Verification items for the finished model (mm, model axes). A direction names the side the tool comes from. Give positions to 0.01 mm unless a question says otherwise; leave off trailing zeros. Loops run counter-clockwise (first coordinate to the right, second up) from the corner with the lowest first, then second, coordinate; pieces in that order, holes last. Notation, with made-up numbers: M 5.25,-30.75 L 59.25,-30.75 A23 ccw 59.25,-6.75 Z; hole C -12.5,-36.75 d5. An arc over 180 degrees is marked long. Use a Markdown table: item, result.
from build123d import *

# Parameters (mm, degrees)
SKETCH1_W           = 88
SKETCH1_H           = 40
BOSS_EXTRUDE1_DEPTH = 3.175
CUT_EXTRUDE1_REACH  = 5.175
SKETCH2_W           = 16
SKETCH2_H           = 3.175
SKETCH2_W_2         = 8
CUT_EXTRUDE2_REACH  = 5.175
SKETCH3_W           = 3.175
SKETCH3_H           = 8
CUT_EXTRUDE3_REACH  = 5.175
SKETCH4_R           = 2.5
CUT_EXTRUDE4_REACH  = 5.175
SKETCH5_R           = 2.5


with BuildPart() as part:
    # Sketch1 → Boss-Extrude1 (new body)
    with BuildSketch(Plane(origin=(0, 0, 0), x_dir=(1, 0, 0), z_dir=(0, 1, 0))):
        with Locations((44, -20)):
            Rectangle(SKETCH1_W, SKETCH1_H)
    extrude(amount=BOSS_EXTRUDE1_DEPTH)

    # Sketch2 → Cut-Extrude1 (cut, up to next)
    with BuildSketch(Plane(origin=(0, 3.175, 0), x_dir=(1, 0, 0), z_dir=(0, 1, 0)), mode=Mode.PRIVATE) as cut_extrude1_sk1:
        with Locations((8, -1.5875)):
            Rectangle(SKETCH2_W, SKETCH2_H)
    cut_extrude1_tool1 = extrude(cut_extrude1_sk1.sketch, amount=-CUT_EXTRUDE1_REACH, mode=Mode.PRIVATE) & part.part
    add(cut_extrude1_tool1.solids().sort_by_distance((8, 3.175, 1.5875))[0], mode=Mode.SUBTRACT)
    # Sketch2 → Cut-Extrude1 (cut, up to next)
    with BuildSketch(Plane(origin=(0, 3.175, 0), x_dir=(1, 0, 0), z_dir=(0, 1, 0)), mode=Mode.PRIVATE) as cut_extrude1_sk2:
        with Locations((44, -1.5875)):
            Rectangle(SKETCH2_W_2, SKETCH2_H)
    cut_extrude1_tool2 = extrude(cut_extrude1_sk2.sketch, amount=-CUT_EXTRUDE1_REACH, mode=Mode.PRIVATE) & part.part
    add(cut_extrude1_tool2.solids().sort_by_distance((44, 3.175, 1.5875))[0], mode=Mode.SUBTRACT)
    # Sketch2 → Cut-Extrude1 (cut, up to next)
    with BuildSketch(Plane(origin=(0, 3.175, 0), x_dir=(1, 0, 0), z_dir=(0, 1, 0)), mode=Mode.PRIVATE) as cut_extrude1_sk3:
        with Locations((60, -1.5875)):
            Rectangle(SKETCH2_W_2, SKETCH2_H)
    cut_extrude1_tool3 = extrude(cut_extrude1_sk3.sketch, amount=-CUT_EXTRUDE1_REACH, mode=Mode.PRIVATE) & part.part
    add(cut_extrude1_tool3.solids().sort_by_distance((60, 3.175, 1.5875))[0], mode=Mode.SUBTRACT)
    # Sketch2 → Cut-Extrude1 (cut, up to next)
    with BuildSketch(Plane(origin=(0, 3.175, 0), x_dir=(1, 0, 0), z_dir=(0, 1, 0)), mode=Mode.PRIVATE) as cut_extrude1_sk4:
        with Locations((80, -1.5875)):
            Rectangle(SKETCH2_W, SKETCH2_H)
    cut_extrude1_tool4 = extrude(cut_extrude1_sk4.sketch, amount=-CUT_EXTRUDE1_REACH, mode=Mode.PRIVATE) & part.part
    add(cut_extrude1_tool4.solids().sort_by_distance((80, 3.175, 1.5875))[0], mode=Mode.SUBTRACT)
    # Sketch2 → Cut-Extrude1 (cut, up to next)
    with BuildSketch(Plane(origin=(0, 3.175, 0), x_dir=(1, 0, 0), z_dir=(0, 1, 0)), mode=Mode.PRIVATE) as cut_extrude1_sk5:
        with Locations((28, -1.5875)):
            Rectangle(SKETCH2_W_2, SKETCH2_H)
    cut_extrude1_tool5 = extrude(cut_extrude1_sk5.sketch, amount=-CUT_EXTRUDE1_REACH, mode=Mode.PRIVATE) & part.part
    add(cut_extrude1_tool5.solids().sort_by_distance((28, 3.175, 1.5875))[0], mode=Mode.SUBTRACT)
    # Sketch2 → Cut-Extrude1 (cut, up to next)
    with BuildSketch(Plane(origin=(0, 3.175, 0), x_dir=(1, 0, 0), z_dir=(0, 1, 0)), mode=Mode.PRIVATE) as cut_extrude1_sk6:
        with Locations((44, -38.4125)):
            Rectangle(SKETCH2_W_2, SKETCH2_H)
    cut_extrude1_tool6 = extrude(cut_extrude1_sk6.sketch, amount=-CUT_EXTRUDE1_REACH, mode=Mode.PRIVATE) & part.part
    add(cut_extrude1_tool6.solids().sort_by_distance((44, 3.175, 38.4125))[0], mode=Mode.SUBTRACT)
    # Sketch2 → Cut-Extrude1 (cut, up to next)
    with BuildSketch(Plane(origin=(0, 3.175, 0), x_dir=(1, 0, 0), z_dir=(0, 1, 0)), mode=Mode.PRIVATE) as cut_extrude1_sk7:
        with Locations((28, -38.4125)):
            Rectangle(SKETCH2_W_2, SKETCH2_H)
    cut_extrude1_tool7 = extrude(cut_extrude1_sk7.sketch, amount=-CUT_EXTRUDE1_REACH, mode=Mode.PRIVATE) & part.part
    add(cut_extrude1_tool7.solids().sort_by_distance((28, 3.175, 38.4125))[0], mode=Mode.SUBTRACT)
    # Sketch2 → Cut-Extrude1 (cut, up to next)
    with BuildSketch(Plane(origin=(0, 3.175, 0), x_dir=(1, 0, 0), z_dir=(0, 1, 0)), mode=Mode.PRIVATE) as cut_extrude1_sk8:
        with Locations((8, -38.4125)):
            Rectangle(SKETCH2_W, SKETCH2_H)
    cut_extrude1_tool8 = extrude(cut_extrude1_sk8.sketch, amount=-CUT_EXTRUDE1_REACH, mode=Mode.PRIVATE) & part.part
    add(cut_extrude1_tool8.solids().sort_by_distance((8, 3.175, 38.4125))[0], mode=Mode.SUBTRACT)
    # Sketch2 → Cut-Extrude1 (cut, up to next)
    with BuildSketch(Plane(origin=(0, 3.175, 0), x_dir=(1, 0, 0), z_dir=(0, 1, 0)), mode=Mode.PRIVATE) as cut_extrude1_sk9:
        with Locations((80, -38.4125)):
            Rectangle(SKETCH2_W, SKETCH2_H)
    cut_extrude1_tool9 = extrude(cut_extrude1_sk9.sketch, amount=-CUT_EXTRUDE1_REACH, mode=Mode.PRIVATE) & part.part
    add(cut_extrude1_tool9.solids().sort_by_distance((80, 3.175, 38.4125))[0], mode=Mode.SUBTRACT)
    # Sketch2 → Cut-Extrude1 (cut, up to next)
    with BuildSketch(Plane(origin=(0, 3.175, 0), x_dir=(1, 0, 0), z_dir=(0, 1, 0)), mode=Mode.PRIVATE) as cut_extrude1_sk10:
        with Locations((60, -38.4125)):
            Rectangle(SKETCH2_W_2, SKETCH2_H)
    cut_extrude1_tool10 = extrude(cut_extrude1_sk10.sketch, amount=-CUT_EXTRUDE1_REACH, mode=Mode.PRIVATE) & part.part
    add(cut_extrude1_tool10.solids().sort_by_distance((60, 3.175, 38.4125))[0], mode=Mode.SUBTRACT)

    # Sketch3 → Cut-Extrude2 (cut, up to next)
    with BuildSketch(Plane(origin=(0, 3.175, 0), x_dir=(1, 0, 0), z_dir=(0, 1, 0)), mode=Mode.PRIVATE) as cut_extrude2_sk1:
        with Locations((1.5875, -28)):
            Rectangle(SKETCH3_W, SKETCH3_H)
    cut_extrude2_tool1 = extrude(cut_extrude2_sk1.sketch, amount=-CUT_EXTRUDE2_REACH, mode=Mode.PRIVATE) & part.part
    add(cut_extrude2_tool1.solids().sort_by_distance((1.5875, 3.175, 28))[0], mode=Mode.SUBTRACT)
    # Sketch3 → Cut-Extrude2 (cut, up to next)
    with BuildSketch(Plane(origin=(0, 3.175, 0), x_dir=(1, 0, 0), z_dir=(0, 1, 0)), mode=Mode.PRIVATE) as cut_extrude2_sk2:
        with Locations((1.5875, -12)):
            Rectangle(SKETCH3_W, SKETCH3_H)
    cut_extrude2_tool2 = extrude(cut_extrude2_sk2.sketch, amount=-CUT_EXTRUDE2_REACH, mode=Mode.PRIVATE) & part.part
    add(cut_extrude2_tool2.solids().sort_by_distance((1.5875, 3.175, 12))[0], mode=Mode.SUBTRACT)
    # Sketch3 → Cut-Extrude2 (cut, up to next)
    with BuildSketch(Plane(origin=(0, 3.175, 0), x_dir=(1, 0, 0), z_dir=(0, 1, 0)), mode=Mode.PRIVATE) as cut_extrude2_sk3:
        with Locations((86.4125, -28)):
            Rectangle(SKETCH3_W, SKETCH3_H)
    cut_extrude2_tool3 = extrude(cut_extrude2_sk3.sketch, amount=-CUT_EXTRUDE2_REACH, mode=Mode.PRIVATE) & part.part
    add(cut_extrude2_tool3.solids().sort_by_distance((86.4125, 3.175, 28))[0], mode=Mode.SUBTRACT)
    # Sketch3 → Cut-Extrude2 (cut, up to next)
    with BuildSketch(Plane(origin=(0, 3.175, 0), x_dir=(1, 0, 0), z_dir=(0, 1, 0)), mode=Mode.PRIVATE) as cut_extrude2_sk4:
        with Locations((86.4125, -12)):
            Rectangle(SKETCH3_W, SKETCH3_H)
    cut_extrude2_tool4 = extrude(cut_extrude2_sk4.sketch, amount=-CUT_EXTRUDE2_REACH, mode=Mode.PRIVATE) & part.part
    add(cut_extrude2_tool4.solids().sort_by_distance((86.4125, 3.175, 12))[0], mode=Mode.SUBTRACT)

    # Sketch4 → Cut-Extrude3 (cut, up to next)
    with BuildSketch(Plane(origin=(0, 3.175, 0), x_dir=(1, 0, 0), z_dir=(0, 1, 0)), mode=Mode.PRIVATE) as cut_extrude3_sk1:
        with Locations((78.41, -28)):
            Circle(SKETCH4_R)
    cut_extrude3_tool1 = extrude(cut_extrude3_sk1.sketch, amount=-CUT_EXTRUDE3_REACH, mode=Mode.PRIVATE) & part.part
    add(cut_extrude3_tool1.solids().sort_by_distance((78.41, 3.175, 28))[0], mode=Mode.SUBTRACT)
    # Sketch4 → Cut-Extrude3 (cut, up to next)
    with BuildSketch(Plane(origin=(0, 3.175, 0), x_dir=(1, 0, 0), z_dir=(0, 1, 0)), mode=Mode.PRIVATE) as cut_extrude3_sk2:
        with Locations((78.41, -12)):
            Circle(SKETCH4_R)
    cut_extrude3_tool2 = extrude(cut_extrude3_sk2.sketch, amount=-CUT_EXTRUDE3_REACH, mode=Mode.PRIVATE) & part.part
    add(cut_extrude3_tool2.solids().sort_by_distance((78.41, 3.175, 12))[0], mode=Mode.SUBTRACT)
    # Sketch4 → Cut-Extrude3 (cut, up to next)
    with BuildSketch(Plane(origin=(0, 3.175, 0), x_dir=(1, 0, 0), z_dir=(0, 1, 0)), mode=Mode.PRIVATE) as cut_extrude3_sk3:
        with Locations((78.41, -20)):
            Circle(SKETCH4_R)
    cut_extrude3_tool3 = extrude(cut_extrude3_sk3.sketch, amount=-CUT_EXTRUDE3_REACH, mode=Mode.PRIVATE) & part.part
    add(cut_extrude3_tool3.solids().sort_by_distance((78.41, 3.175, 20))[0], mode=Mode.SUBTRACT)

    # Sketch5 → Cut-Extrude4 (cut, up to next)
    with BuildSketch(Plane(origin=(0, 3.175, 0), x_dir=(1, 0, 0), z_dir=(0, 1, 0)), mode=Mode.PRIVATE) as cut_extrude4_sk1:
        with Locations((10.5, -12)):
            Circle(SKETCH5_R)
    cut_extrude4_tool1 = extrude(cut_extrude4_sk1.sketch, amount=-CUT_EXTRUDE4_REACH, mode=Mode.PRIVATE) & part.part
    add(cut_extrude4_tool1.solids().sort_by_distance((10.5, 3.175, 12))[0], mode=Mode.SUBTRACT)
    # Sketch5 → Cut-Extrude4 (cut, up to next)
    with BuildSketch(Plane(origin=(0, 3.175, 0), x_dir=(1, 0, 0), z_dir=(0, 1, 0)), mode=Mode.PRIVATE) as cut_extrude4_sk2:
        with Locations((10.5, -28)):
            Circle(SKETCH5_R)
    cut_extrude4_tool2 = extrude(cut_extrude4_sk2.sketch, amount=-CUT_EXTRUDE4_REACH, mode=Mode.PRIVATE) & part.part
    add(cut_extrude4_tool2.solids().sort_by_distance((10.5, 3.175, 28))[0], mode=Mode.SUBTRACT)
    # Sketch5 → Cut-Extrude4 (cut, up to next)
    with BuildSketch(Plane(origin=(0, 3.175, 0), x_dir=(1, 0, 0), z_dir=(0, 1, 0)), mode=Mode.PRIVATE) as cut_extrude4_sk3:
        with BuildLine():
            Line((9, -16.5), (12, -16.5))
            ThreePointArc((12, -16.5), (12.707106781, -16.792893219), (13, -17.5))
            Line((13, -17.5), (13, -22.5))
            ThreePointArc((13, -22.5), (12.707106781, -23.207106781), (12, -23.5))
            Line((12, -23.5), (9, -23.5))
            ThreePointArc((9, -23.5), (8.292893219, -23.207106781), (8, -22.5))
            Line((8, -22.5), (8, -17.5))
            ThreePointArc((8, -17.5), (8.292893219, -16.792893219), (9, -16.5))
        make_face()
    cut_extrude4_tool3 = extrude(cut_extrude4_sk3.sketch, amount=-CUT_EXTRUDE4_REACH, mode=Mode.PRIVATE) & part.part
    add(cut_extrude4_tool3.solids().sort_by_distance((10.5, 3.175, 20))[0], mode=Mode.SUBTRACT)


solid = part.part
(1) Cross-section at A-A on z = 28. Record the cut outline in (x, y) (3 decimals), then the cut area to 3 significant figures.
Results below:
| item | result |
|---|---|
| outline | M 3.175,0 L 8,0 L 8,3.175 L 3.175,3.175 Z; M 13,0 L 75.91,0 L 75.91,3.175 L 13,3.175 Z; M 80.91,0 L 84.825,0 L 84.825,3.175 L 80.91,3.175 Z |
| area | 227 mm^2 |
(2) Draft check along X on faces 1 (the flat face through (44, 2, 3.175)), 2 (the flat face through (64, 2, 2)), 3 (the flat face through (20, 2, 40)), 4 (the flat face through (0, 2, 6)). Enter one of: +X half, -X half, draft (parallel to the pull), parting line (faces both ways), or undercut.
Results below:
| item | result |
|---|---|
| face 1 | undercut |
| face 2 | undercut |
| face 3 | draft |
| face 4 | -X half |
(3) Cross-section at C-C on y = 1.8. State how many separate pieces and enclosed holes the cut face has, then the cut area to 3 significant figures.
Results below:
| item | result |
|---|---|
| separate pieces | 1 |
| enclosed holes | 6 |
| area | 2,930 mm^2 |
(4) Material ranges on line 1 (Z direction, x = 10.5, y = 2.45) (3 decimals); line 2 (Z direction, x = 78.41, y = 1.1) (3 decimals); line 3 (X direction, y = 0.65, z = 28) (3 decimals), recorded low to high.
Results below:
| item | result |
|---|---|
| line 1 | 3.175 to 9.5, 14.5 to 16.5, 23.5 to 25.5, 30.5 to 36.825 |
| line 2 | 3.175 to 9.5, 14.5 to 17.5, 22.5 to 25.5, 30.5 to 36.825 |
| line 3 | 3.175 to 8, 13 to 75.91, 80.91 to 84.825 |
(5) Set-up check for faces 5 (the flat face through (13, 2, 20)), 6 (the flat face through (2, 2, 24)), 7 (the flat face through (40, 2, 38)), 8 (the flat face through (32, 2, 2)), 9 (the flat face through (8, 2, 36.825)): record each of +Z, -Z, +X, -X, +Y, -Y from which the full face is reachable in a straight line by a thin tool's end or side.
Results below:
| item | result |
|---|---|
| face 5 | +Y, -Y |
| face 6 | -X, +Y, -Y |
| face 7 | +Z, +Y, -Y |
| face 8 | -Z, +Y, -Y |
| face 9 | +Z, -X, +Y, -Y |
(6) Cross-section at D-D on z = 20. Record the cut outline in (x, y) (3 decimals).
Results below:
| item | result |
|---|---|
| outline | M 0,0 L 8,0 L 8,3.175 L 0,3.175 Z; M 13,0 L 75.91,0 L 75.91,3.175 L 13,3.175 Z; M 80.91,0 L 88,0 L 88,3.175 L 80.91,3.175 Z |
(7) Gauge pin test, flat ends, axial feed: P1, Ø1, axis at x = 7.5, y = 1.5, coming from the +Z side (3 decimals); P2, Ø1.6, axis at x = 86, y = 2, coming from the -Z side (3 decimals); P3, Ø4.5, axis at x = 10.5, z = 12, coming from the -Y side; P4, Ø1, axis at y = 2.5, z = 1, coming from the -X side. Record the tip position at first contact, or that the pin passes through.
Results below:
| item | result |
|---|---|
| P1 | z = 36.825 |
| P2 | z = 3.175 |
| P3 | through |
| P4 | x = 16 |
(8) Cross-section at B-B on x = 78.41. Record the cut outline in (y, z) (3 decimals).
Results below:
| item | result |
|---|---|
| outline | M 0,3.175 L 3.175,3.175 L 3.175,9.5 L 0,9.5 Z; M 0,14.5 L 3.175,14.5 L 3.175,17.5 L 0,17.5 Z; M 0,22.5 L 3.175,22.5 L 3.175,25.5 L 0,25.5 Z; M 0,30.5 L 3.175,30.5 L 3.175,36.825 L 0,36.825 Z |
